Autodesk Inventor part; units mm, degrees
ref_plane "YZ Plane" through (0, 0, 0) normal (1, 0, 0) x (0, 1, 0)
ref_plane "XZ Plane" through (0, 0, 0) normal (0, 1, 0) x (-1, 0, 0)
ref_plane "XY Plane" through (0, 0, 0) normal (0, 0, 1) x (1, 0, 0)
sketch "Эскиз1" plane through (0, 0, 0) normal (0, 0, 1) x (1, 0, 0)
  line L0 (0, 0) -> (34.5, 0)
  line L1 (34.5, 0) -> (34.5, 9.5)
  line L2 (34.5, 9.5) -> (0, 9.5)
  line L3 (0, 9.5) -> (0, 0)
  line L4 (3, 9.5) -> (3, 0)
  line L5 (31.5, 9.5) -> (31.5, 0)
  line L6 (3, 3) -> (31.5, 3)
  dimension "d0" = 34.5
  dimension "d1" = 9.5
  dimension "d2" = 3
  dimension "d3" = 3
  dimension "d4" = 3
extrude "Выдавливание1" add sketch "Эскиз1" along normal blind 295 contours L3 L2 L4 L0 | L4 L6 L5 L0 | L5 L2 L1 L0
fillet "Сопряжение1" radius 2 4 edges at (3, 3, 147.5) (31.5, 3, 147.5) (34.5, 9.5, 147.5) (0, 9.5, 147.5)
sketch "Эскиз2" plane through (0, 0, 0) normal (0, -1, 0) x (1, 0, 0)
  line L0 (0, 0) -> (34.5, 0)
  line L1 (34.5, 0) -> (34.5, 295)
  line L2 (0, 295) -> (34.5, 295)
  line L3 (0, 0) -> (0, 295)
  line L4 (17.25, 295) -> (17.25, 0)
  line L5 (22.25, 217) -> (12.25, 217)
  line L6 (12.25, 217) -> (12.25, 254)
  line L7 (12.25, 254) -> (22.25, 254)
  line L8 (22.25, 254) -> (22.25, 217)
  line L9 (22.25, 217) -> (12.25, 254) construction
  line L10 (12.25, 217) -> (22.25, 254) construction
  line L11 (12.25, 111.5) -> (22.25, 111.5)
  line L12 (22.25, 111.5) -> (22.25, 148.5)
  line L13 (22.25, 148.5) -> (12.25, 148.5)
  line L14 (12.25, 148.5) -> (12.25, 111.5)
  line L15 (12.25, 111.5) -> (22.25, 148.5) construction
  line L16 (22.25, 111.5) -> (12.25, 148.5) construction
  line L17 (22.25, 37.5) -> (12.25, 37.5)
  line L18 (12.25, 37.5) -> (12.25, 54.5)
  line L19 (12.25, 54.5) -> (22.25, 54.5)
  line L20 (22.25, 54.5) -> (22.25, 37.5)
  line L21 (22.25, 37.5) -> (12.25, 54.5) construction
  line L22 (12.25, 37.5) -> (22.25, 54.5) construction
  point P0 (17.25, 235.5)
  point P1 (17.25, 130)
  point P2 (17.25, 46)
  dimension "d8" = 10
  dimension "d9" = 37
  dimension "d10" = 41
  dimension "d11" = 10
  dimension "d12" = 37
  dimension "d13" = 68.5
  dimension "d14" = 10
  dimension "d15" = 17
  dimension "d16" = 57
extrude "Выдавливание2" cut sketch "Эскиз2" against normal blind 295 contours L17 L18 L19 L4 | L4 L19 L20 L17 | L7 L8 L5 L4 | L4 L5 L6 L7 | L11 L14 L13 L4 | L4 L13 L12 L11
fillet "Сопряжение2" radius 2 12 edges at (12.25, 1.5, 148.5) (12.25, 1.5, 111.5) (22.25, 1.5, 111.5) (22.25, 1.5, 148.5) (22.25, 1.5, 54.5) (22.25, 1.5, 37.5) (12.25, 1.5, 54.5) (12.25, 1.5, 37.5) (12.25, 1.5, 217) (12.25, 1.5, 254) (22.25, 1.5, 254) (22.25, 1.5, 217)
properties part number "2 часть направляшки"
Could you check a few things on this model? Use its own coordinates, in mm. A direction names the side the tool comes from. Give positions to 0.01 mm unless a question says otherwise; leave off trailing zeros. Order: outer loops, then holes, each group sorted by start corner. A loop starts at its lowest first (then second) coordinate and runs counter-clockwise, first axis right, second up.
Item 1: If we section it at B-B, the plane y = 1.5: Write out the boundary of the cut face in (x, z).
Item 2: If we mould it in two halves opening along X, with no side actions, what happens to faces 3 (the face through (25, 0, 145)), 4 (the face through (0, 4, 145)), 5 (the face through (23, 3, 145))? For each: pulls with the +X half, pulls with the -X half, needs draft (parallel to the pull), parting line crosses it, or undercut.
Item 3: I need wall thicknesses on line 1 (Z direction, x = 14, y = 1.25); line 2 (X direction, y = 7.5, z = 136.5); line 3 (X direction, y = 1, z = 221.5). Which ranges of each line are inside material? Lowest first, please.
Item 4: I'm going to push flat-ended pins straight in: pin 1 (19.5 mm diameter, centred on x = 20.5, z = 159, fed in from +Y); pin 2 (12 mm diameter, centred on x = 21.5, z = 64.5, fed in from +Y); pin 3 (2 mm diameter, centred on y = 8, z = 214, fed in from +X). Where does each tip first touch, or does it pass through?
Item 5: If we section it at C-C, the plane z = 116.5: Write out the boundary of the cut face in (x, y), plus the area to 4 significant figures.
Item 6: For faces 1 (the face through (3, 7, 145)), 2 (the face through (17, 2.7, 0)), which set-ups out of +Z, -Z, +X, -X, +Y, -Y let a thin tool reach every point of the face, with its end or its side?
Item 7: If we section it at D-D, the plane z = 19: Write out the boundary of the cut face in (x, y), plus the area to 4 significant figures.
Item 8: If we section it at A-A, the plane x = 17.5: Write out the boundary of the cut face in (y, z).
Values:
1. outline: (0, 0) - (34.5, 0) - (34.5, 295) - (0, 295) - close; hole (12.25, 39.5) arc R2 ccw to (14.25, 37.5) - (20.25, 37.5) arc R2 ccw to (22.25, 39.5) - (22.25, 52.5) arc R2 ccw to (20.25, 54.5) - (14.25, 54.5) arc R2 ccw to (12.25, 52.5) - close; hole (12.25, 113.5) arc R2 ccw to (14.25, 111.5) - (20.25, 111.5) arc R2 ccw to (22.25, 113.5) - (22.25, 146.5) arc R2 ccw to (20.25, 148.5) - (14.25, 148.5) arc R2 ccw to (12.25, 146.5) - close; hole (12.25, 219) arc R2 ccw to (14.25, 217) - (20.25, 217) arc R2 ccw to (22.25, 219) - (22.25, 252) arc R2 ccw to (20.25, 254) - (14.25, 254) arc R2 ccw to (12.25, 252) - close
2. face 3: needs draft
2. face 4: pulls with the -X half
2. face 5: undercut
3. line 1: z = 0 to 37.52, 54.48 to 111.52, 148.48 to 217.02, 253.98 to 295
3. line 2: x = 0 to 3, 31.5 to 34.5
3. line 3: x = 0 to 12.25, 22.25 to 34.5
4. pin 1: stops at y = 3.15
4. pin 2: stops at y = 3
4. pin 3: stops at x = 34.5
5. outline: (0, 0) - (12.25, 0) - (12.25, 3) - (5, 3) arc R2 cw to (3, 5) - (3, 9.5) - (2, 9.5) arc R2 ccw to (0, 7.5) - close; (22.25, 0) - (34.5, 0) - (34.5, 7.5) arc R2 ccw to (32.5, 9.5) - (31.5, 9.5) - (31.5, 5) arc R2 cw to (29.5, 3) - (22.25, 3) - close
5. area: 112.5 mm2
6. face 1: +Z, -Z, +Y
6. face 2: -Z, +X, -X, +Y, -Y
7. outline: (0, 0) - (34.5, 0) - (34.5, 7.5) arc R2 ccw to (32.5, 9.5) - (31.5, 9.5) - (31.5, 5) arc R2 cw to (29.5, 3) - (5, 3) arc R2 cw to (3, 5) - (3, 9.5) - (2, 9.5) arc R2 ccw to (0, 7.5) - close
7. area: 142.5 mm2
8. outline: (0, 0) - (3, 0) - (3, 37.5) - (0, 37.5) - close; (0, 54.5) - (3, 54.5) - (3, 111.5) - (0, 111.5) - close; (0, 148.5) - (3, 148.5) - (3, 217) - (0, 217) - close; (0, 254) - (3, 254) - (3, 295) - (0, 295) - close
